Model file for the job. Use its own axes, mm. A direction names the side the tool comes from. Round coordinates to 2 decimals unless told otherwise and drop trailing zeros. Order: outer loops, then holes, each group sorted by start corner. A loop starts at its lowest first (then second) coordinate and runs counter-clockwise, first axis right, second up. Notation, with made-up numbers: (64, 10) -> (100, 10) arc R22 ccw to (100, 20) -> close; hole circle Ø4 at (55.5, -12.5). An arc over 180 degrees is marked (long way). Use CSV: the item, a comma, the result in double quotes.
```python
from build123d import *

# Parameters (mm, degrees)
BOSS_EXTRUDE1_DEPTH       = 3.175
F_4_CLEARANCE_HOLE1_D     = 2.9464
F_4_CLEARANCE_HOLE1_DEPTH = 3.302
F_4_CLEARANCE_HOLE1_TIP   = 0.885187864
CUT_EXTRUDE1_REACH        = 5.175
SKETCH4_R                 = 4.7625
BOSS_EXTRUDE2_DEPTH       = 3.175


with BuildPart() as part:
    # Sketch1 → Boss-Extrude1 (new body)
    with BuildSketch(Plane.XY):
        Polygon((7.9375, -3.175), (10.8966, -3.175), (10.8966, 3.175), (-10.8966, 3.175), (-10.8966, -3.175), (-7.9375, -3.175), (-7.9375, -22.225), (-10.8966, -22.225), (-10.8966, -28.575), (10.8966, -28.575), (10.8966, -22.225), (7.9375, -22.225), align=None)
    extrude(amount=BOSS_EXTRUDE1_DEPTH)

    # #4 Clearance Hole1
    with Locations(Plane.XY.offset(3.175)):
        with Locations((0, 0), (0, -25.4)):
            Hole(F_4_CLEARANCE_HOLE1_D / 2, depth=F_4_CLEARANCE_HOLE1_DEPTH)
            with Locations((0, 0, -(F_4_CLEARANCE_HOLE1_DEPTH + F_4_CLEARANCE_HOLE1_TIP / 2))):  # 118° drill point
                Cone(0, F_4_CLEARANCE_HOLE1_D / 2, F_4_CLEARANCE_HOLE1_TIP, mode=Mode.SUBTRACT)

    # Sketch4 → Cut-Extrude1 (cut, up to next)
    with BuildSketch(Plane.XY.offset(3.175), mode=Mode.PRIVATE) as cut_extrude1_sk1:
        with Locations((0, -12.7)):
            Circle(SKETCH4_R)
    cut_extrude1_tool1 = extrude(cut_extrude1_sk1.sketch, amount=-CUT_EXTRUDE1_REACH, mode=Mode.PRIVATE) & part.part
    add(cut_extrude1_tool1.solids().sort_by_distance((0, -12.7, 3.175))[0], mode=Mode.SUBTRACT)

    # Sketch5 → Boss-Extrude2 (add)
    with BuildSketch(Plane.XY.offset(3.175)):
        Polygon((-10.8966, -3.175), (-10.8966, -22.225), (-10.8966, -28.575), (-18, -28.575), (-18, -16.002), (-15, -16.002), (-15, -9.398), (-18, -9.398), (-18, 3.175), (-10.8966, 3.175), align=None)
    extrude(amount=-BOSS_EXTRUDE2_DEPTH)


solid = part.part
```
Q1. Cut at A-A (y = -12.7). Give the cut face in (x, z) (1 decimal), plus the area to 3 significant figures.
From the geometry:
outline,"(-15, 0) -> (-10.9, 0) -> (-10.9, 3.2) -> (-15, 3.2) -> close; (-7.9, 0) -> (-4.8, 0) -> (-4.8, 3.2) -> (-7.9, 3.2) -> close; (4.8, 0) -> (7.9, 0) -> (7.9, 3.2) -> (4.8, 3.2) -> close"
area,"33.2 mm²"
Q2. Which spindle directions (+Z, -Z, +X, -X, +Y, -Y) get a long thin tool onto all of the face, cutting with end or side? Do faces 5 (the flat face through (-7, -12, 3.175)), 6 (the flat face through (-10.897, -13, 2)), 7 (the flat face through (9, -3.175, 2)), 8 (the flat face through (-15, -13, 2)). Say none if no direction does.
From the geometry:
face 5,"+Z, +X, -X, +Y, -Y"
face 6,"+Z, -Z"
face 7,"+Z, -Z, +X"
face 8,"+Z, -Z, -X"
Q3. Mould opens along X. For faces 1 (the flat face through (-3, -28.575, 2)), 2 (the flat face through (-9, -3.175, 2)), 3 (the flat face through (-18, -3, 2)), 4 (the cylindrical face through (3, -9, 2)) say: +X half, -X half, draft (parallel to the pull), parting line (faces both ways), or undercut.
From the geometry:
face 1,"draft"
face 2,"undercut"
face 3,"-X half"
face 4,"undercut"
Q4. Pin check, flat tips, straight feed: pin 1 (1.8 mm diameter, centred on x = 0, y = -25.4, fed in from +Z); pin 2 (1.5 mm diameter, centred on y = -5, z = 1.5, fed in from +X). Stop position of each tip, or through.
From the geometry:
pin 1,"passes through"
pin 2,"stops at x = 7.94"
Q5. Cut at D-D (y = -25.4). Give the cut face in (x, z) (3 decimals).
From the geometry:
outline,"(-18, 0) -> (-1.473, 0) -> (-1.473, 3.175) -> (-18, 3.175) -> close; (1.473, 0) -> (10.897, 0) -> (10.897, 3.175) -> (1.473, 3.175) -> close"
Q6. Cut at C-C (x = 0). Give the cut face in (y, z) (1 decimal), plus the area to 3 significant figures.
From the geometry:
outline,"(-28.6, 0) -> (-26.9, 0) -> (-26.9, 3.2) -> (-28.6, 3.2) -> close; (-23.9, 0) -> (-17.5, 0) -> (-17.5, 3.2) -> (-23.9, 3.2) -> close; (-7.9, 0) -> (-1.5, 0) -> (-1.5, 3.2) -> (-7.9, 3.2) -> close; (1.5, 0) -> (3.2, 0) -> (3.2, 3.2) -> (1.5, 3.2) -> close"
area,"51.9 mm²"
Q7. Probe line 1 along Y through (x, z) = (0, 1.9) (1 decimal); line 2 along X through (y, z) = (-19.5, 1.2); line 3 along X through (y, z) = (-16.5, 2.8). List the from-to ranges inside material, lowest first.
From the geometry:
line 1,"y = -28.6 to -26.9, -23.9 to -17.5, -7.9 to -1.5, 1.5 to 3.2"
line 2,"x = -18 to -10.9, -7.94 to 7.94"
line 3,"x = -18 to -10.9, -7.94 to -2.87, 2.87 to 7.94"
Q8. Cut at B-B (z = 1.45). Give the cut face in (x, y) (1 decimal), plus the area to 3 significant figures.
From the geometry:
outline,"(-18, -28.6) -> (10.9, -28.6) -> (10.9, -22.2) -> (7.9, -22.2) -> (7.9, -3.2) -> (10.9, -3.2) -> (10.9, 3.2) -> (-18, 3.2) -> (-18, -9.4) -> (-15, -9.4) -> (-15, -16) -> (-18, -16) -> close; hole (-10.9, -22.2) -> (-7.9, -22.2) -> (-7.9, -3.2) -> (-10.9, -3.2) -> close; hole circle Ø9.5 at (0, -12.7); hole circle Ø2.9 at (0, -25.4); hole circle Ø2.9 at (0, 0)"
area,"700 mm²"
